The drawing under review shows one solid part. Ordinate dimensions are in mm from its lowest x, y, z. Coordinates: 2 decimals unless noted, no trailing zeros. Write each loop counter-clockwise with the first axis right and the second up, starting at its lowest first coordinate (ties: lowest second). Pieces come first, ordered by that corner, then holes.
1) Add section B-B, the plane y = 20.5. State the section outline as (x, z) points (1 decimal), then the cut area to 3 significant figures.
2) For line 1 (Y direction, x = 17, z = 52); line 2 (X direction, y = 29.5, z = 47.5) (1 decimal); line 3 (Y direction, x = 27, z = 21.5), list the stretches that pass through material, from the lowest coordinate up.
3) For P1, Ø8, axis at x = 12.5, z = 35, coming from the -Y side; P2, Ø4, axis at x = 35, y = 32.5, coming from the -Z side (1 decimal); P3, Ø8, axis at y = 39, z = 22.5, coming from the +X side; P4, Ø10, axis at x = 35.5, z = 36.5, coming from the +Y side, all flat-tipped, find the tip position at first contact; note any pin that passes through.
4) Mouldability with a two-part tool opening along X and no side actions: class the marked faces 1, 2 and 3 as released by +X, released by -X, zero draft, split by the parting line, or undercut.
5) Add section A-A, the plane y = 40.5. State the section outline as (x, z) points (1 decimal), then the cut area to 3 significant figures.
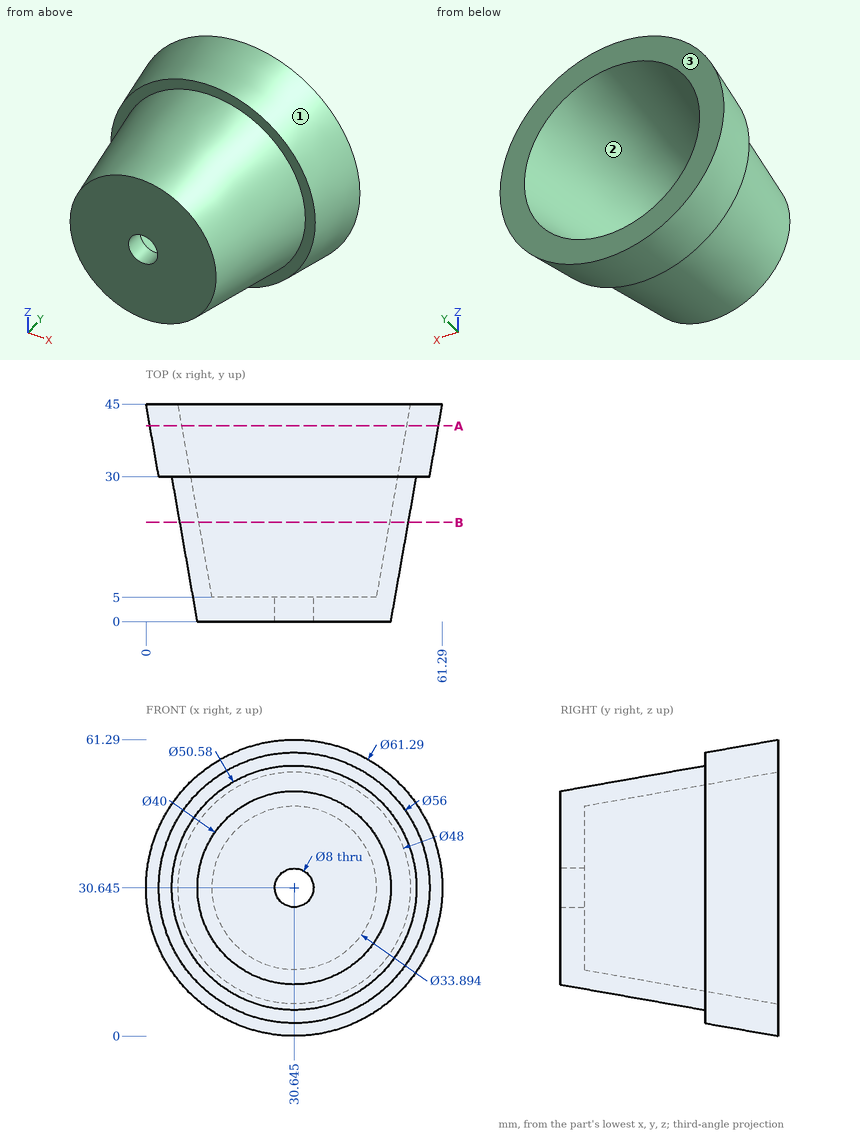
Geometry results:
1. outline: circle Ø47.2 at (30.6, 30.6); hole circle Ø39.4 at (30.6, 30.6)
1. area: 535 mm2
2. line 1: y = 30 to 45
2. line 2: x = 11.9 to 17.7, 43.6 to 49.4
2. line 3: y = 0 to 5
3. P1: stops at y = 0
3. P2: stops at z = 2.1
3. P3: stops at x = 60.26
3. P4: stops at y = 5
4. face 1: split by the parting line
4. face 2: undercut
4. face 3: zero draft
5. outline: circle Ø59.7 at (30.6, 30.6); hole circle Ø46.4 at (30.6, 30.6)
5. area: 1,110 mm2
